from build123d import *

# Parameters (mm, degrees)
SKETCH1_W           = 25
SKETCH1_H           = 48
BOSS_EXTRUDE1_DEPTH = 10
BOSS_EXTRUDE2_DEPTH = 48
SKETCH4_W           = 17.037497091
SKETCH4_H           = 48
CUT_EXTRUDE1_DEPTH  = 48
SKETCH5_W           = 20
SKETCH5_H           = 40
CUT_EXTRUDE2_DEPTH  = 3


with BuildPart() as part:
    # Sketch1 → Boss-Extrude1 (new body)
    with BuildSketch(Plane.XY):
        with Locations((12.5, 24)):
            Rectangle(SKETCH1_W, SKETCH1_H)
    extrude(amount=BOSS_EXTRUDE1_DEPTH)

    # Sketch3 → Boss-Extrude2 (add)
    with BuildSketch(Plane(origin=(0, 48, 0), x_dir=(1, 0, 0), z_dir=(0, 1, 0))):
        with BuildLine():
            Line((0, -1.170858034), (0, -10))
            Line((0, -10), (25, -10))
            Line((25, -10), (25, -1.170858034))
            ThreePointArc((25, -1.170858034), (12.5, 0), (0, -1.170858034))
        make_face()
    extrude(amount=BOSS_EXTRUDE2_DEPTH)

    # Sketch4 → Cut-Extrude1 (cut)
    with BuildSketch(Plane(origin=(25, 0, 0), x_dir=(0, 0, -1), z_dir=(1, 0, 0))):
        with Locations((-8.518748546, 24)):
            Rectangle(SKETCH4_W, SKETCH4_H)
    extrude(amount=-CUT_EXTRUDE1_DEPTH, mode=Mode.SUBTRACT)

    # Sketch5 → Cut-Extrude2 (cut)
    with BuildSketch(Plane.XY.offset(10)):
        with Locations((12.5, 72)):
            Rectangle(SKETCH5_W, SKETCH5_H)
    extrude(amount=-CUT_EXTRUDE2_DEPTH, mode=Mode.SUBTRACT)


solid = part.part
Work out the finished part from the listing and answer in its coordinate system (mm). A direction names the side the tool comes from. Give positions to 0.01 mm unless a question says otherwise; leave off trailing zeros. Loops run counter-clockwise (first coordinate to the right, second up) from the corner with the lowest first, then second, coordinate; pieces in that order, holes last. Notation, with made-up numbers: (48.5, 57.5) -> (95.5, 57.5) arc R26 ccw to (95.5, 82.5) -> close; hole circle Ø2 at (85.5, 68). An arc over 180 degrees is marked (long way). Use a Markdown table: item, result. Add a question column.
1) Consider line 1 along Y through (x, z) = (13.5, 8.25); line 2 along X through (y, z) = (55, 9); line 3 along Z through (x, y) = (13.25, 71). Determine where each line is inside the solid, lowest interval first.
2) Which of the six approach directions +Z, -Z, +X, -X, +Y, -Y give full straight-line access (tool end or side, diameter ignored) to faces 4 (the flat face through (25, 72, 6)), 5 (the flat face through (2.5, 72, 9))?
3) For a pull along Y with two mould halves and no side action, classify faces 1 (the cylindrical face through (13, 72, 0)), 2 (the flat face through (13, 48, 5)), 3 (the flat face through (12, 52, 9)) as +Y half, -Y half, draft (parallel to the pull), parting line (faces both ways), or undercut.
4) The part is cut by section B-B, the plane y = 76.5. Determine the outline of the cut face in (x, z).
5) The part is cut by section C-C, the plane x = 5.25. Determine the outline of the cut face in (y, z).
6) This flat-tipped pin is pushed along its axis until it touches: P1, Ø10, axis at x = 11.5, y = 77, coming from the +Z side. Where does it stop, or does it pass through?
7) The part is cut by section A-A, the plane z = 8.5. Determine the outline of the cut face in (x, y), plus the area to 3 significant figures.
8) The part is cut by section D-D, the plane y = 93.5. Determine the outline of the cut face in (x, z).
Reported:
| question | item | result |
|---|---|---|
| 1 | line 1 | y = 48 to 52, 92 to 96 |
| 1 | line 2 | x = 0 to 2.5, 22.5 to 25 |
| 1 | line 3 | z = 0 to 7 |
| 2 | face 4 | +Z, -Z, +X, +Y, -Y |
| 2 | face 5 | +Z |
| 3 | face 1 | draft |
| 3 | face 2 | -Y half |
| 3 | face 3 | undercut |
| 4 | outline | (0, 1.17) arc R67.31 ccw to (25, 1.17) -> (25, 10) -> (22.5, 10) -> (22.5, 7) -> (2.5, 7) -> (2.5, 10) -> (0, 10) -> close |
| 5 | outline | (48, 0.39) -> (96, 0.39) -> (96, 10) -> (92, 10) -> (92, 7) -> (52, 7) -> (52, 10) -> (48, 10) -> close |
| 6 | P1 | stops at z = 7 |
| 7 | outline | (0, 48) -> (25, 48) -> (25, 96) -> (0, 96) -> close; hole (2.5, 52) -> (22.5, 52) -> (22.5, 92) -> (2.5, 92) -> close |
| 7 | area | 400 mm^2 |
| 8 | outline | (0, 1.17) arc R67.31 ccw to (25, 1.17) -> (25, 10) -> (0, 10) -> close |
